from build123d import *

# Parameters (mm, degrees)
BASE_FLANGE1_DEPTH       = 2
SKETCHED_BEND1_OUTLINE_W = 2
SKETCHED_BEND1_OUTLINE_H = 35
SKETCHED_BEND1_DEPTH     = 44.40715449
SKETCHED_START           = 45.98523449
SKETCHED_BEND1_2_DEPTH   = 0.01096
SKETCHED_START_2         = 43.99619449
SKETCHED_BEND1_3_DEPTH   = 4
SKETCHED_START_3         = -17.5
SKETCHED_BEND1_4_DEPTH   = 35
SKETCH7_R                = 2
CUT_EXTRUDE1_DEPTH       = 10


with BuildPart() as part:
    # Base-Flange1: sheet metal written as solids
    # Sketch1 → Base-Flange1 (new body)
    with BuildSketch(Plane(origin=(0, 0, 0), x_dir=(1, 0, 0), z_dir=(0, 1, 0))):
        with BuildLine():
            Line((0, 16.5), (0, 5.83))
            ThreePointArc((0, 5.83), (0.292893219, 5.122893219), (1, 4.83))
            Line((1, 4.83), (10.67, 4.83))
            ThreePointArc((10.67, 4.83), (12, 3.5), (10.67, 2.17))
            Line((10.67, 2.17), (1, 2.17))
            ThreePointArc((1, 2.17), (0.292893219, 1.877106781), (0, 1.17))
            Line((0, 1.17), (0, -1.17))
            ThreePointArc((0, -1.17), (0.292893219, -1.877106781), (1, -2.17))
            Line((1, -2.17), (10.67, -2.17))
            ThreePointArc((10.67, -2.17), (12, -3.5), (10.67, -4.83))
            Line((10.67, -4.83), (1, -4.83))
            ThreePointArc((1, -4.83), (0.292893219, -5.122893219), (0, -5.83))
            Line((0, -5.83), (0, -16.5))
            ThreePointArc((0, -16.5), (0.292893219, -17.207106781), (1, -17.5))
            Line((1, -17.5), (49, -17.5))
            ThreePointArc((49, -17.5), (49.707106781, -17.207106781), (50, -16.5))
            Line((50, -16.5), (50, -6.17))
            ThreePointArc((50, -6.17), (50.292893219, -5.462893219), (51, -5.17))
            Line((51, -5.17), (57, -5.17))
            ThreePointArc((57, -5.17), (57.707106781, -4.877106781), (58, -4.17))
            Line((58, -4.17), (58, -1.83))
            ThreePointArc((58, -1.83), (57.707106781, -1.122893219), (57, -0.83))
            Line((57, -0.83), (51, -0.83))
            ThreePointArc((51, -0.83), (50.292893219, -0.537106781), (50, 0.17))
            Line((50, 0.17), (50, 16.5))
            ThreePointArc((50, 16.5), (49.707106781, 17.207106781), (49, 17.5))
            Line((49, 17.5), (1, 17.5))
            ThreePointArc((1, 17.5), (0.292893219, 17.207106781), (0, 16.5))
        make_face()
    extrude(amount=-BASE_FLANGE1_DEPTH)

    # Sketched Bend1: read off the stored shape, not the designer's step
    # Sketched Bend1 outline → Sketched Bend1 (cut)
    with BuildSketch(Plane.YZ):
        with Locations((-1, 0)):
            Rectangle(SKETCHED_BEND1_OUTLINE_W, SKETCHED_BEND1_OUTLINE_H)
    extrude(amount=SKETCHED_BEND1_DEPTH, mode=Mode.SUBTRACT)

    # Sketched Bend1 2 outline → Sketched Bend1 2 (add)
    with BuildSketch(Plane.YZ.offset(SKETCHED_START)):
        with BuildLine():
            Line((0, -17.5), (44.28380551, -17.5))
            ThreePointArc((44.28380551, -17.5), (44.990912291, -17.207106781), (45.28380551, -16.5))
            Line((45.28380551, -16.5), (45.28380551, -5.83))
            ThreePointArc((45.28380551, -5.83), (44.990912291, -5.122893219), (44.28380551, -4.83))
            Line((44.28380551, -4.83), (34.61380551, -4.83))
            ThreePointArc((34.61380551, -4.83), (33.28380551, -3.5), (34.61380551, -2.17))
            Line((34.61380551, -2.17), (44.28380551, -2.17))
            ThreePointArc((44.28380551, -2.17), (44.990912291, -1.877106781), (45.28380551, -1.17))
            Line((45.28380551, -1.17), (45.28380551, 1.17))
            ThreePointArc((45.28380551, 1.17), (44.990912291, 1.877106781), (44.28380551, 2.17))
            Line((44.28380551, 2.17), (34.61380551, 2.17))
            ThreePointArc((34.61380551, 2.17), (33.28380551, 3.5), (34.61380551, 4.83))
            Line((34.61380551, 4.83), (44.28380551, 4.83))
            ThreePointArc((44.28380551, 4.83), (44.990912291, 5.122893219), (45.28380551, 5.83))
            Line((45.28380551, 5.83), (45.28380551, 16.5))
            ThreePointArc((45.28380551, 16.5), (44.990912291, 17.207106781), (44.28380551, 17.5))
            Line((44.28380551, 17.5), (0, 17.5))
            Line((0, 17.5), (0, -17.5))
        make_face()
    extrude(amount=SKETCHED_BEND1_2_DEPTH)

    # Sketched Bend1 3 outline → Sketched Bend1 3 (add)
    with BuildSketch(Plane.YZ.offset(SKETCHED_START_2)):
        with BuildLine():
            Line((0, -17.5), (44.28380551, -17.5))
            ThreePointArc((44.28380551, -17.5), (44.990912291, -17.207106781), (45.28380551, -16.5))
            Line((45.28380551, -16.5), (45.28380551, -5.83))
            ThreePointArc((45.28380551, -5.83), (44.990912291, -5.122893219), (44.28380551, -4.83))
            Line((44.28380551, -4.83), (34.61380551, -4.83))
            ThreePointArc((34.61380551, -4.83), (33.28380551, -3.5), (34.61380551, -2.17))
            Line((34.61380551, -2.17), (44.28380551, -2.17))
            ThreePointArc((44.28380551, -2.17), (44.990912291, -1.877106781), (45.28380551, -1.17))
            Line((45.28380551, -1.17), (45.28380551, 1.17))
            ThreePointArc((45.28380551, 1.17), (44.990912291, 1.877106781), (44.28380551, 2.17))
            Line((44.28380551, 2.17), (34.61380551, 2.17))
            ThreePointArc((34.61380551, 2.17), (33.28380551, 3.5), (34.61380551, 4.83))
            Line((34.61380551, 4.83), (44.28380551, 4.83))
            ThreePointArc((44.28380551, 4.83), (44.990912291, 5.122893219), (45.28380551, 5.83))
            Line((45.28380551, 5.83), (45.28380551, 16.5))
            ThreePointArc((45.28380551, 16.5), (44.990912291, 17.207106781), (44.28380551, 17.5))
            Line((44.28380551, 17.5), (0, 17.5))
            Line((0, 17.5), (0, -17.5))
        make_face()
    extrude(amount=SKETCHED_BEND1_3_DEPTH)

    # Sketched Bend1 4 outline → Sketched Bend1 4 (cut)
    with BuildSketch(Plane.XY.offset(SKETCHED_START_3)):
        with BuildLine():
            Line((47.99619449, 45.28380551), (45.99619449, 45.28380551))
            Line((45.99619449, 45.28380551), (45.99619449, 2))
            ThreePointArc((45.99619449, 2), (46.581980928, 0.585786438), (47.99619449, 0))
            Line((47.99619449, 0), (47.99619449, 45.28380551))
        make_face()
        with BuildLine():
            ThreePointArc((47.99619449, -2), (45.167767365, -0.828427125), (43.99619449, 2))
            Line((43.99619449, 2), (43.99619449, 0))
            Line((43.99619449, 0), (44.40715449, 0))
            Line((44.40715449, 0), (44.40715449, -2))
            Line((44.40715449, -2), (47.99619449, -2))
        make_face()
    extrude(amount=SKETCHED_BEND1_4_DEPTH, mode=Mode.SUBTRACT)

    # Sketch7 → Cut-Extrude1 (cut)
    with BuildSketch(Plane.ZY.offset(-43.99619449)):
        with Locations(Location((0, 6, 0), (0, 0, 270))):
            Circle(SKETCH7_R)
    extrude(amount=-CUT_EXTRUDE1_DEPTH, mode=Mode.SUBTRACT)


solid = part.part
Here's how the part is built. I have some questions about the finished solid (model axes, mm). A direction names the side the tool comes from. Round coordinates to 2 decimals unless told otherwise and drop trailing zeros. Order: outer loops, then holes, each group sorted by start corner. A loop starts at its lowest first (then second) coordinate and runs counter-clockwise, first axis right, second up. Notation, with made-up numbers: (9, 36.5) -> (48, 36.5) arc R22 ccw to (48, 53.5) -> close; hole circle Ø4 at (77.5, 25). An arc over 180 degrees is marked (long way). Use CSV: the item, a comma, the result in double quotes.
1. I'm going to push flat-ended pins straight in: P1, Ø6.5, axis at y = 6, z = 0, coming from the -X side; P2, Ø0.6, axis at x = 55, y = -1, coming from the -Z side; P3, Ø1.5, axis at x = 52, z = -6, coming from the -Y side; P4, Ø1, axis at y = -0.5, z = -8.5, coming from the +X side. Where does each tip first touch, or does it pass through?
Recorded:
P1,"stops at x = 44"
P2,"stops at z = 0.83"
P3,"passes through"
P4,"stops at x = 50"
2. Thinking about a two-plate mould opening in Z: for faces 1 (the face through (50.301, -0.986, 0.545)), 2 (the face through (45, 7.6, -1.2)), 3 (the face through (50.285, -0.986, 5.471)), which applies, pulls with the +Z half, pulls with the -Z half, needs draft (parallel to the pull), parting line crosses it, or undercut?
Recorded:
face 1,"pulls with the -Z half"
face 2,"undercut"
face 3,"pulls with the +Z half"
3. I want a section at A-A on y = 6. List the corners of the cut face in (x, z) for me.
Recorded:
outline,"(44, -17.5) -> (46, -17.5) -> (46, -2) -> (44, -2) -> close; (44, 2) -> (46, 2) -> (46, 17.5) -> (44, 17.5) -> close"
4. I want a section at C-C on x = 45.25. List the corners of the cut face in (y, z) for me.
Recorded:
outline,"(-0.91, -17.5) -> (44.28, -17.5) arc R1 ccw to (45.28, -16.5) -> (45.28, -5.83) arc R1 ccw to (44.28, -4.83) -> (34.61, -4.83) arc R1.33 cw to (34.61, -2.17) -> (44.28, -2.17) arc R1 ccw to (45.28, -1.17) -> (45.28, 1.17) arc R1 ccw to (44.28, 2.17) -> (34.61, 2.17) arc R1.33 cw to (34.61, 4.83) -> (44.28, 4.83) arc R1 ccw to (45.28, 5.83) -> (45.28, 16.5) arc R1 ccw to (44.28, 17.5) -> (-0.91, 17.5) -> close; hole circle Ø4 at (6, 0)"
5. I need wall thicknesses on line 1 along Z through (x, y) = (44.85, 6); line 2 along X through (y, z) = (2.5, 12.5); line 3 along Y through (x, z) = (49, 2). Which ranges of each line are inside material? Lowest first, please.
Recorded:
line 1,"z = -17.5 to -2, 2 to 17.5"
line 2,"x = 44 to 46"
line 3,"y = -2 to 0"
6. I want a section at D-D on x = 51.75. List the corners of the cut face in (y, z) for me.
Recorded:
outline,"(-2, 0.83) -> (0, 0.83) -> (0, 5.17) -> (-2, 5.17) -> close"
7. I want a section at B-B on z = 3.5. List the corners of the cut face in (x, y) for me.
Recorded:
outline,"(44, 2) arc R4 ccw to (48, -2) -> (58, -2) -> (58, 0) -> (48, 0) arc R2 cw to (46, 2) -> (46, 33.28) -> (44, 33.28) -> close"
8. Which directions (+Z, -Z, +X, -X, +Y, -Y) give clear straight access to the entire face, cutting with the end or side of a thin tool? Please do faces 4 (the face through (51, 0, 3)), 5 (the face through (51, -2, 3)), 6 (the face through (44.98, 45, -5.13)).
Recorded:
face 4,"+Z, -Z, +X, +Y"
face 5,"+Z, -Z, +X, -X, -Y"
face 6,"+X, -X, +Y"
